Can you work these out from the drawing? Everything is in mm from the part's minimum corner. A direction names the side the tool comes from. Coordinates: 2 decimals unless noted, no trailing zeros. Loops run counter-clockwise (first coordinate to the right, second up) from the corner with the lowest first, then second, coordinate; pieces in that order, holes last. Notation, with made-up numbers: (68, 82) -> (93, 82) arc R26 ccw to (93, 104) -> close; hole circle Ø10 at (-4, 20). An arc over 180 degrees is marked (long way). Put each result on its own line as item: value. Start each with the question number.
Item 1: Will these pins go through, and if not, where does the flat tip stop? P1, Ø2.5, axis at x = 5, z = 5, coming from the +Y side; P2, Ø2, axis at x = 32, z = 3.5, coming from the +Y side; P3, Ø1, axis at y = 28, z = 4.5, coming from the -X side; P4, Ø5, axis at x = 29, z = 5, coming from the -Y side.
Item 2: If we section it at B-B on z = 5: Please give me the cut outline in (x, y) (1 decimal), plus the area to 3 significant figures.
Item 3: If we section it at C-C on x = 5: Please give me the cut outline in (y, z).
Item 4: If we section it at D-D on x = 30: Please give me the cut outline in (y, z), plus the area to 3 significant figures.
Item 5: For the marked faces 1 and 2, which set-ups out of +Z, -Z, +X, -X, +Y, -Y let a thin tool reach every point of the face, with its end or its side?
Item 6: If we section it at A-A on y = 3.1: Please give me the cut outline in (x, z).
Item 7: We'd pull the mould along Y, two halves only. Please class the marked faces 3, 4 and 5: pulls with the +Y half, pulls with the -Y half, needs draft (parallel to the pull), parting line crosses it, or undercut.
Item 8: Please list where these lines run through material, in increasing order: L1, parallel to Y at x = 43.5, z = 3.25 (1 decimal); L2, parallel to Z at x = 30, y = 2; L3, parallel to Y at x = 47.5, z = 8.25 (1 decimal). Write a range as from..to.
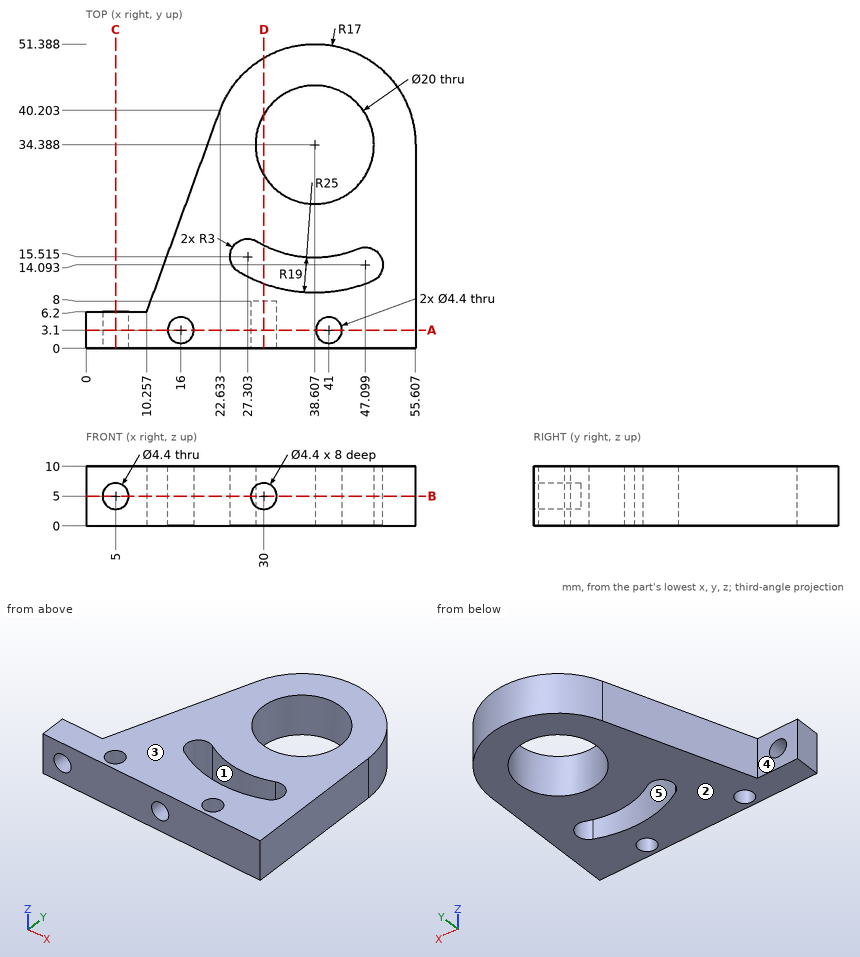
Solutions:
1. P1: through
1. P2: y = 50.44
1. P3: x = 18.01
1. P4: y = 0
2. outline: (0, 0) -> (2.8, 0) -> (2.8, 6.2) -> (0, 6.2) -> close; (7.2, 0) -> (27.8, 0) -> (27.8, 8) -> (32.2, 8) -> (32.2, 0) -> (55.6, 0) -> (55.6, 34.4) arc R17 ccw to (22.6, 40.2) -> (10.3, 6.2) -> (7.2, 6.2) -> close; hole circle Ø4.4 at (16, 3.1); hole (25.8, 12.9) arc R25 ccw to (48.3, 11.3) arc R3 ccw to (45.9, 16.9) arc R19 cw to (28.8, 18.1) arc R3 ccw to start; hole circle Ø20 at (38.6, 34.4); hole circle Ø4.4 at (41, 3.1)
2. area: 1,380 mm^2
3. outline: (0, 0) -> (6.2, 0) -> (6.2, 2.8) -> (0, 2.8) -> close; (0, 7.2) -> (6.2, 7.2) -> (6.2, 10) -> (0, 10) -> close
4. outline: (0, 0) -> (10.92, 0) -> (10.92, 10) -> (0, 10) -> (0, 7.2) -> (8, 7.2) -> (8, 2.8) -> (0, 2.8) -> close; (17.45, 0) -> (29.3, 0) -> (29.3, 10) -> (17.45, 10) -> close; (39.48, 0) -> (49.05, 0) -> (49.05, 10) -> (39.48, 10) -> close
4. area: 288 mm^2
5. face 1: +Z, -Z
5. face 2: -Z, +X, -X, +Y, -Y
6. outline: (0, 0) -> (13.8, 0) -> (13.8, 10) -> (0, 10) -> close; (18.2, 0) -> (38.8, 0) -> (38.8, 10) -> (18.2, 10) -> close; (43.2, 0) -> (55.61, 0) -> (55.61, 10) -> (43.2, 10) -> close; hole circle Ø4.4 at (5, 5); hole circle Ø4.4 at (30, 5)
7. face 3: needs draft
7. face 4: pulls with the +Y half
7. face 5: undercut
8. L1: 0..9.9, 16..25.7, 43.1..50.7
8. L2: 0..2.8, 7.2..10
8. L3: 0..11, 17.1..29.8, 39..48.9
